Autodesk Inventor part; units mm, degrees
ref_plane "YZ Plane" through (0, 0, 0) normal (1, 0, 0) x (0, 1, 0)
ref_plane "XZ Plane" through (0, 0, 0) normal (0, 1, 0) x (-1, 0, 0)
ref_plane "XY Plane" through (0, 0, 0) normal (0, 0, 1) x (1, 0, 0)
sketch "Skizze1" plane through (0, 0, 0) normal (0, 0, 1) x (1, 0, 0)
  circle A0 centre (0, 0) radius 8.5
  dimension "d0" = 17
extrude "Extrusion1" add sketch "Skizze1" against normal mid plane 4.5
sketch "Skizze2" plane through (0, 0, -2.25) normal (0, 0, -1) x (-1, 0, 0)
  circle A0 centre (0, 0) radius 7.5
  dimension "d3" = 15
extrude "Extrusion2" cut sketch "Skizze2" against normal blind 1
sketch "Skizze3" plane through (0, 0, 2.25) normal (0, 0, 1) x (1, 0, 0)
  circle A0 centre (0, 0) radius 3.5
  dimension "d6" = 7
extrude "Extrusion3" cut sketch "Skizze3" against normal blind 1
sketch "Skizze4" plane through (0, 0, 1.25) normal (0, 0, 1) x (1, 0, 0)
  circle A0 centre (0, 0) radius 1.6
  dimension "d9" = 3.2
extrude "Extrusion4" cut sketch "Skizze4" against normal up to surface (2.5 mm away)
properties part number "_3D-Druck"
Source: CAD feature listing. Evaluate the final solid. Frame: model axes, mm. A direction names the side the tool comes from. Coordinates: 2 decimals unless noted, no trailing zeros. Write each loop counter-clockwise with the first axis right and the second up, starting at its lowest first coordinate (ties: lowest second). Pieces come first, ordered by that corner, then holes. Notation, with made-up numbers: (80, 82) - (91, 82) arc R14 ccw to (91, 103) - close; hole circle Ø9 at (-1, -36.5). An arc over 180 degrees is marked (long way). Answer as a JSON object with one key per item and string values.
Q1. Section query C-C, the plane z = -0.15. Output: boundary loops of the cut face in (x, y), plus the area to 3 significant figures.
Ans:
{"outline": "circle Ø17 at (0, 0); hole circle Ø3.2 at (0, 0)", "area": "219 mm2"}
Q2. Section query D-D, the plane x = 2.25. Output: boundary loops of the cut face in (y, z).
Ans:
{"outline": "(-8.2, -2.25) - (-7.15, -2.25) - (-7.15, -1.25) - (7.15, -1.25) - (7.15, -2.25) - (8.2, -2.25) - (8.2, 2.25) - (2.68, 2.25) - (2.68, 1.25) - (-2.68, 1.25) - (-2.68, 2.25) - (-8.2, 2.25) - close"}
Q3. First-contact query: pin 1 Ø4 at (x, y) = (0, 0) entering from +Z; pin 2 Ø6 at (x, y) = (-3.5, 1) entering from -Z; pin 3 Ø1.5 at (y, z) = (1.5, -1.5) entering from -X; pin 4 Ø8 at (x, y) = (-1.5, -1.5) entering from +Z. Flat tips, straight axial feed; report the tip coordinate or a pass-through.
Ans:
{"pin 1": "stops at z = 1.25", "pin 2": "stops at z = -1.25", "pin 3": "stops at x = -8.47", "pin 4": "stops at z = 2.25"}
Q4. Material intervals for line 1 (Y direction, x = 0, z = -0.3); line 2 (Y direction, x = 0, z = -1.6); line 3 (Z direction, x = 3.5, y = -3.75), sorted ascending. Write a range as [from, to].
Ans:
{"line 1": "y = [-8.5, -1.6], [1.6, 8.5]", "line 2": "y = [-8.5, -7.5], [7.5, 8.5]", "line 3": "z = [-1.25, 2.25]"}
Q5. Set-up query: faces 5 (the flat face through (0, 2, -1.25)), 6 (the flat face through (0, -8, -2.25)). Return all of +Z, -Z, +X, -X, +Y, -Y with unobstructed straight access to the full face (end or side cutting, diameter ignored); none if empty.
Ans:
{"face 5": "-Z", "face 6": "-Z, +X, -X, +Y, -Y"}
Q6. Section query A-A, the plane x = 0. Output: boundary loops of the cut face in (y, z).
Ans:
{"outline": "(-8.5, -2.25) - (-7.5, -2.25) - (-7.5, -1.25) - (-1.6, -1.25) - (-1.6, 1.25) - (-3.5, 1.25) - (-3.5, 2.25) - (-8.5, 2.25) - close; (1.6, -1.25) - (7.5, -1.25) - (7.5, -2.25) - (8.5, -2.25) - (8.5, 2.25) - (3.5, 2.25) - (3.5, 1.25) - (1.6, 1.25) - close"}
Q7. Draft query along X for faces 1 (the cylindrical face through (4.57, 7.167, 0.031)), 2 (the flat face through (4, 0, 2.25)), 3 (the cylindrical face through (3.233, -1.341, 1.757)), 4 (the flat face through (1, -2, 1.25)). Return one class per face: released by +X, released by -X, zero draft, split by the parting line, or undercut.
Ans:
{"face 1": "split by the parting line", "face 2": "zero draft", "face 3": "undercut", "face 4": "undercut"}
